Can you work these out from the drawing? Everything is in mm from the part's minimum corner. Round coordinates to 2 decimals unless told otherwise and drop trailing zeros. Write each loop counter-clockwise with the first axis right and the second up, starting at its lowest first coordinate (ties: lowest second). Pieces come first, ordered by that corner, then holes. Notation, with made-up numbers: (17.25, -34.75) - (61.25, -34.75) arc R31 cw to (61.25, -0.75) - close; hole circle Ø6 at (37.25, 17). An arc over 180 degrees is marked (long way). Write each question's results on one line, items separated by ' | '. Start each with the question number.
(1) For P1, Ø6, axis at x = 76.5, z = 17.5, coming from the -Y side; P2, Ø6.5, axis at x = 88.5, z = 20, coming from the +Y side, each with a flat end and sliding along its axis, tell me the tip position at first contact or that it passes through.
(2) Imagine slicing it at C-C on x = 18.5. Write out the boundary of the cut face in (y, z), then the cut area to 3 significant figures.
(3) Thinking about a two-plate mould opening in X: for the marked faces 1, 2, 3 and 4, which applies, +X half, -X half, draft (parallel to the pull), parting line (faces both ways), or undercut?
(4) Imagine slicing it at B-B on z = 5. Write out the boundary of the cut face in (x, y), then the cut area to 3 significant figures.
(5) Imagine slicing it at A-A on x = 88.5. Write out the boundary of the cut face in (y, z), then the cut area to 3 significant figures.
(6) Please list where these lines run through material, in increasing order: line 1 (Z direction, x = 6.5, y = 5); line 2 (Z direction, x = 76.5, y = 1.5); line 3 (Z direction, x = 47.5, y = 4.25). Write a range as [from, to].
(7) Imagine slicing it at D-D on y = 3.5. Write out the boundary of the cut face in (x, z).
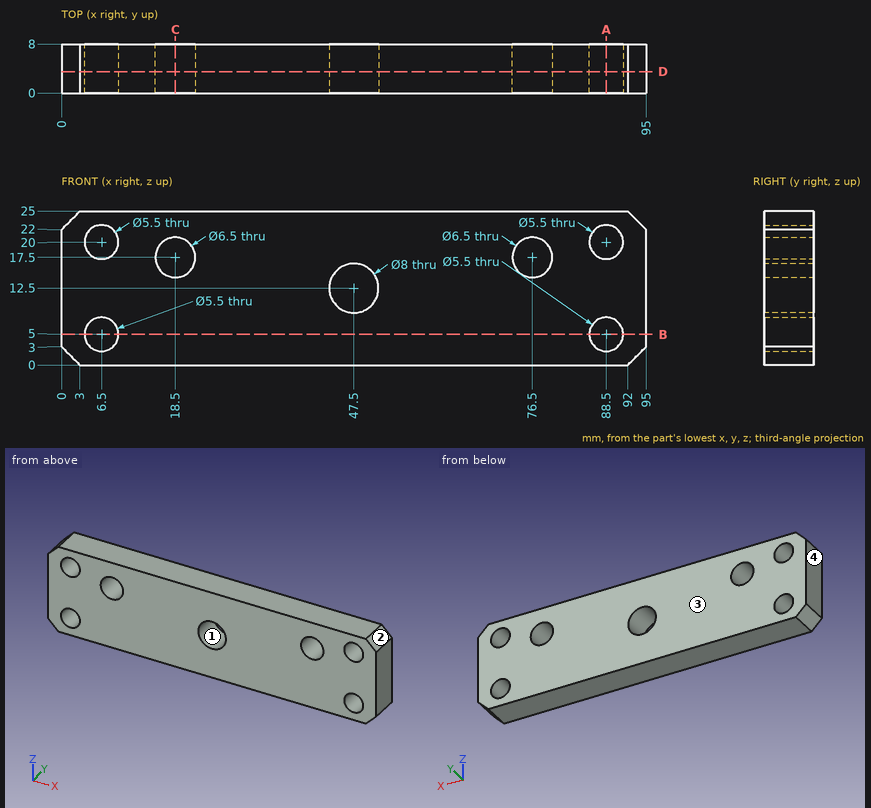
Response:
1) P1: through | P2: y = 8
2) outline: (0, 0) - (8, 0) - (8, 14.25) - (0, 14.25) - close; (0, 20.75) - (8, 20.75) - (8, 25) - (0, 25) - close | area: 148 mm²
3) face 1: undercut | face 2: +X half | face 3: draft | face 4: -X half
4) outline: (0, 0) - (3.75, 0) - (3.75, 8) - (0, 8) - close; (9.25, 0) - (85.75, 0) - (85.75, 8) - (9.25, 8) - close; (91.25, 0) - (95, 0) - (95, 8) - (91.25, 8) - close | area: 672 mm²
5) outline: (0, 0) - (8, 0) - (8, 2.25) - (0, 2.25) - close; (0, 7.75) - (8, 7.75) - (8, 17.25) - (0, 17.25) - close; (0, 22.75) - (8, 22.75) - (8, 25) - (0, 25) - close | area: 112 mm²
6) line 1: [0, 2.25], [7.75, 17.25], [22.75, 25] | line 2: [0, 14.25], [20.75, 25] | line 3: [0, 8.5], [16.5, 25]
7) outline: (0, 3) - (3, 0) - (92, 0) - (95, 3) - (95, 22) - (92, 25) - (3, 25) - (0, 22) - close; hole circle Ø5.5 at (6.5, 5); hole circle Ø5.5 at (6.5, 20); hole circle Ø6.5 at (18.5, 17.5); hole circle Ø8 at (47.5, 12.5); hole circle Ø6.5 at (76.5, 17.5); hole circle Ø5.5 at (88.5, 5); hole circle Ø5.5 at (88.5, 20)
